Geometry check sheet. Reference: the model listing, model coordinates, mm. A direction names the side the tool comes from. Round coordinates to 2 decimals unless told otherwise and drop trailing zeros. Order: outer loops, then holes, each group sorted by start corner. A loop starts at its lowest first (then second) coordinate and runs counter-clockwise, first axis right, second up. Notation, with made-up numbers: M 15,48 L 25,48 A17 cw 25,56 Z; hole C -28.5,-36 d7. An arc over 180 degrees is marked long. Answer as a JSON object with one key per item and string values. Group by question number.
```python
from build123d import *

# Parameters (mm, degrees)
SKETCH1_W                      = 5.475
SKETCH1_H                      = 7
SKETCH2_R                      = 4.5
BOSS_EXTRUDE1_DEPTH            = 3.9
F_5_0_5_DIAMETER_HOLE1_D       = 5
F_5_0_5_DIAMETER_HOLE1_DEPTH   = 10.9
F_2_5_2_5_DIAMETER_HOLE1_D     = 2.5
F_2_5_2_5_DIAMETER_HOLE1_DEPTH = 3.309936491
SKETCH7_W                      = 1.25
SKETCH7_H                      = 3.960443852


with BuildPart() as part:
    # Sketch1 → Revolve1 (revolve)
    with BuildSketch(Plane.XY.offset(-56.4)):
        with Locations((78.2375, 52.926431985)):
            Rectangle(SKETCH1_W, SKETCH1_H)
    revolve(axis=Axis((75.5, 56.426431985, -56.4), (0, -1, 0)))

    # Sketch2 → Boss-Extrude1 (add)
    with BuildSketch(Plane.XZ.offset(-49.426431985)):
        with Locations((75.5, -56.4)):
            Circle(SKETCH2_R)
    extrude(amount=BOSS_EXTRUDE1_DEPTH)

    # Ø5.0 (5) Diameter Hole1
    with Locations(Plane(origin=(0, 56.426431985, 0), x_dir=(1, 0, 0), z_dir=(0, 1, 0))):
        with Locations((75.5, 56.4)):
            Hole(F_5_0_5_DIAMETER_HOLE1_D / 2, depth=F_5_0_5_DIAMETER_HOLE1_DEPTH)

    # Ø2.5 (2.5) Diameter Hole1
    with Locations(Plane.ZY.offset(-77.665063509)):
        with Locations((-56.4, 47.476431985)):
            Hole(F_2_5_2_5_DIAMETER_HOLE1_D / 2, depth=F_2_5_2_5_DIAMETER_HOLE1_DEPTH)

    # Sketch7 → Ø2.5 (2.5) Diameter Hole2 (revolve, cut)
    with BuildSketch(Plane(origin=(74.761000333, 47.459423849, -54.885443852), x_dir=(0, 1, 0), z_dir=(1, 0, 0))):
        with Locations((0.625, 1.980221926)):
            Rectangle(SKETCH7_W, SKETCH7_H)
    revolve(axis=Axis((74.761000333, 47.459423849, -61.235443852), (0, 0, 1)), mode=Mode.SUBTRACT)


solid = part.part
```
1) Sectioned sample at C-C (z = -58.5). Record the boundary of the cut face in (x, y).
2) Sectioned sample at D-D (y = 52.5). Record the boundary of the cut face in (x, z) (3 decimals), then the cut area to 3 significant figures.
3) Go/stop test with flat-tipped pins: P1, Ø3, axis at x = 75.5, z = -56.4, coming from the +Y side; P2, Ø2, axis at x = 73, y = 53, coming from the -Z side; P3, Ø3, axis at y = 50, z = -60.5, coming from the -X side; P4, Ø2, axis at y = 47.48, z = -56.4, coming from the +X side. Record where each tip stops, or that it passes through.
4) Set-up check for faces 1 (the flat face through (77.4, 45.526, -58.3)), 2 (the cylindrical face through (77.58, 47.5, -60.39)), 3 (the cylindrical face through (78.849, 46.716, -55.408)): record each of +Z, -Z, +X, -X, +Y, -Y from which the full face is reachable in a straight line by a thin tool's end or side.
5) Thickness scan on line 1 along Y through (x, z) = (79, -56.4); line 2 along Z through (x, y) = (75.5, 52.25) (3 decimals); line 3 along Y through (x, z) = (76.75, -52). Record the ranges inside material, lowest first. Write a range as [from, to].
6) Sectioned sample at B-B (x = 74.25). Record the boundary of the cut face in (y, z), then the cut area to 3 significant figures.
7) Sectioned sample at A-A (z = -56.4). Record the boundary of the cut face in (x, y) (3 decimals).
8) Release check for a two-part mould opening along Y. For faces 4 (the cylindrical face through (73.52, 47.3, -53.04)), 5 (the flat face through (73, 56.426, -58)), 6 (the flat face through (77, 49.426, -61)) record: +Y half, -Y half, draft (parallel to the pull), parting line (faces both ways), or undercut.
Final values:
{
 "1": {"outline": "M 70.44,49.43 L 71.52,49.43 L 71.52,45.53 L 74.14,45.53 L 74.14,56.43 L 70.44,56.43 Z; M 76.86,45.53 L 79.48,45.53 L 79.48,49.43 L 80.56,49.43 L 80.56,56.43 L 76.86,56.43 Z"},
 "2": {"outline": "C 75.5,-56.4 d10.95; hole C 75.5,-56.4 d5", "area": "74.5 mm^2"},
 "3": {"P1": "passes through", "P2": "stops at z = -61.67", "P3": "stops at x = 70.68", "P4": "stops at x = 73.21"},
 "4": {"face 1": "+Z, -Z, +X, -X, -Y", "face 2": "-Y", "face 3": "+X"},
 "5": {"line 1": "y = [45.53, 46.23], [48.73, 56.43]", "line 2": "z = [-61.875, -58.9], [-53.9, -50.925]", "line 3": "y = [49.43, 56.43]"},
 "6": {"outline": "M 45.53,-60.72 L 49.43,-60.72 L 49.43,-61.73 L 56.43,-61.73 L 56.43,-58.57 L 45.53,-58.57 Z; M 45.53,-54.23 L 46.32,-54.23 L 46.32,-52.08 L 45.53,-52.08 Z; M 48.6,-54.23 L 56.43,-54.23 L 56.43,-51.07 L 49.43,-51.07 L 49.43,-52.08 L 48.6,-52.08 Z", "area": "56.2 mm^2"},
 "7": {"outline": "M 70.025,49.426 L 71,49.426 L 71,45.526 L 73,45.526 L 73,56.426 L 70.025,56.426 Z; M 78,45.526 L 80,45.526 L 80,46.226 L 78,46.226 Z; M 78,48.726 L 80,48.726 L 80,49.426 L 80.975,49.426 L 80.975,56.426 L 78,56.426 Z"},
 "8": {"face 4": "undercut", "face 5": "+Y half", "face 6": "-Y half"}
}
